Build history of the part. All positions in model axes, mm. Give positions to 0.01 mm unless a question says otherwise; leave off trailing zeros. Write each loop counter-clockwise with the first axis right and the second up, starting at its lowest first coordinate (ties: lowest second). Pieces come first, ordered by that corner, then holes. Notation, with made-up numbers: (-28, 69) -> (-22, 69) arc R16 cw to (-22, 87) -> close; hole circle Ø8 at (-35, 83). An arc over 180 degrees is marked (long way). Write item = value, one per line. Start each with the question number.
Q1. Wall check: line 1 (Z direction, x = 1.65, y = 12.7); line 2 (Y direction, x = 0.55, z = 23); line 3 (Z direction, x = 1.5, y = 45.72). Give the ranges that are in metal, low to high.
Q2. Mould opens along Z. For faces 1 (the face through (2, 55, 38.1)), 2 (the face through (0, 53, 19)), 3 (the face through (1.5, 13.62, 16.82)) say: pulls with the +Z half, pulls with the -Z half, needs draft (parallel to the pull), parting line crosses it, or undercut.
Q3. Drop a flat-ended pin along its axis: P1, Ø1, axis at y = 22.5, z = 6.5, coming from the -X side. Give the stop position or say it passes through.
Q4. Saw through at D-D, the plane z = 19.05. List the corners of the cut face in (x, y).
Q5. Saw through at B-B, the plane x = 2.15. List the corners of the cut face in (y, z).
Q6. Saw through at A-A, the plane z = 6.35. List the corners of the cut face in (x, y).
Q7. Saw through at C-C, the plane y = 45.72. List the corners of the cut face in (x, z).
Autodesk Fusion 360 part; units mm, degrees
sketch "Sketch1" plane through (0, 0, 0) normal (1, 0, 0) x (0, 1, 0)
  line L0 (0, 0) -> (107.95, 0)
  line L1 (107.95, 0) -> (107.95, 38.1)
  line L2 (107.95, 38.1) -> (0, 38.1)
  line L3 (0, 38.1) -> (0, 0)
  dimension "d1" = 38.1
  dimension "d2" = 107.95
extrude "Extrude1" add sketch "Sketch1" along normal blind 3.048
sketch "Sketch2" plane through (3.048, 0, 0) normal (1, 0, 0) x (0, 1, 0)
  line L0 (0, 38.1) -> (0, 0)
  line L1 (0, 0) -> (107.95, 0)
  line L2 (107.95, 0) -> (107.95, 38.1)
  line L3 (107.95, 38.1) -> (0, 38.1)
  line L4 (-12.7, 0) -> (-12.7, 19.05)
  line L5 (0, -12.7) -> (25.4, -12.7)
  line L6 (25.4, -25.4) -> (31.75, -25.4)
  line L7 (33.02, -38.1) -> (45.72, -38.1)
  line L8 (45.72, -50.8) -> (58.42, -50.8)
  line L9 (58.42, -50.8) -> (58.42, -38.1)
  line L10 (58.42, -38.1) -> (71.12, -38.1)
  line L11 (71.12, -38.1) -> (71.12, -50.8)
  line L12 (71.12, -50.8) -> (83.82, -50.8)
  line L13 (83.82, -50.8) -> (83.82, -38.1)
  line L14 (83.82, -38.1) -> (96.52, -38.1)
  line L15 (96.52, -38.1) -> (96.52, -50.8)
  line L16 (96.52, -50.8) -> (109.22, -50.8)
  line L17 (109.22, -50.8) -> (109.22, -38.1)
  line L18 (-12.7, 19.05) -> (121.92, 19.05)
  circle A0 centre (45.72, 19.05) radius 4.826
  dimension "d5" = 19.05
  dimension "d6" = 6.35
  dimension "d7" = 9.652
hole "Hole1" at (3.048, 45.72, 19.05) direction (-1, 0, 0) diameter 9.652 depth 40.64 tip angle 118
sketch "Sketch3" plane through (3.048, 0, 0) normal (1, 0, 0) x (0, 1, 0)
  circle A0 centre (45.72, 19.05) radius 4.826
  line L0 (0, 38.1) -> (0, 0)
  line L1 (0, 0) -> (107.95, 0)
  line L2 (107.95, 0) -> (107.95, 38.1)
  line L3 (107.95, 38.1) -> (0, 38.1)
  line L4 (111.76, 0) -> (111.76, 19.05)
  circle A1 centre (95.25, 19.0673) radius 4.826
  dimension "d16" = 9.652
hole "Hole2" at (3.048, 95.25, 19.0673) direction (-1, 0, 0) diameter 9.652 depth 40.64 tip angle 118
sketch "Sketch4" plane through (3.048, 0, 0) normal (1, 0, 0) x (0, 1, 0)
  circle A0 centre (95.25, 19.0673) radius 4.826
  circle A1 centre (45.72, 19.05) radius 4.826
  line L0 (0, 38.1) -> (0, 0)
  line L1 (0, 0) -> (107.95, 0)
  line L2 (107.95, 0) -> (107.95, 38.1)
  line L3 (107.95, 38.1) -> (0, 38.1)
  line L4 (12.7, -55.88) -> (0, -55.88)
  line L5 (0, -55.88) -> (0, 45.72)
  line L6 (12.7, 0) -> (-25.4, 0)
  line L7 (0, 0) -> (12.7, 0)
  line L8 (12.7, 0) -> (12.7, 6.35)
  line L9 (12.7, 6.35) -> (0, 6.35)
  line L10 (0, 6.35) -> (0, 0)
  dimension "d22" = 12.7
  dimension "d23" = 6.35
hole "Hole3" at (3.048, 12.7, 6.35) direction (-1, 0, 0) diameter 4.826 depth 40.64 tip angle 118
sketch "Sketch5" plane through (3.048, 0, 0) normal (1, 0, 0) x (0, 1, 0)
  circle A0 centre (12.7, 6.35) radius 2.413
  circle A1 centre (95.25, 19.0673) radius 4.826
  circle A2 centre (45.72, 19.05) radius 4.826
  line L0 (0, 38.1) -> (0, 0)
  line L1 (0, 0) -> (107.95, 0)
  line L2 (107.95, 0) -> (107.95, 38.1)
  line L3 (107.95, 38.1) -> (0, 38.1)
  line L4 (0, 38.1) -> (12.7, 38.1)
  line L5 (12.7, 38.1) -> (12.7, 31.75)
  line L6 (12.7, 31.75) -> (0, 31.75)
  line L7 (0, 31.75) -> (0, 38.1)
  dimension "d27" = 12.7
  dimension "d28" = 6.35
hole "Hole4" at (3.048, 12.7, 31.75) direction (-1, 0, 0) diameter 4.826 depth 40.64 tip angle 118
sketch "Sketch6" plane through (3.048, 0, 0) normal (1, 0, 0) x (0, 1, 0)
  circle A0 centre (12.7, 31.75) radius 2.413
  circle A1 centre (12.7, 6.35) radius 2.413
  circle A2 centre (95.25, 19.0673) radius 4.826
  circle A3 centre (45.72, 19.05) radius 4.826
  line L0 (0, 38.1) -> (0, 0)
  line L1 (0, 0) -> (107.95, 0)
  line L2 (107.95, 0) -> (107.95, 38.1)
  line L3 (107.95, 38.1) -> (0, 38.1)
  line L4 (0, 0) -> (12.7, 0)
  line L5 (12.7, 0) -> (12.7, 19.05)
  line L6 (12.7, 19.05) -> (0, 19.05)
  line L7 (0, 19.05) -> (0, 0)
  dimension "d32" = 12.7
  dimension "d33" = 19.05
hole "Hole5" at (3.048, 12.7, 19.05) direction (-1, 0, 0) diameter 4.826 depth 40.64 tip angle 118
Report:
q1.line_1 = 0 to 3.94, 8.76 to 16.64, 21.46 to 29.34, 34.16 to 38.1
q1.line_2 = 0 to 42.95, 48.49 to 92.45, 98.05 to 107.95
q1.line_3 = 0 to 14.22, 23.88 to 38.1
q2.face_1 = pulls with the +Z half
q2.face_2 = needs draft
q2.face_3 = undercut
q3.P1 = 0
q4.outline = (0, 0) -> (3.05, 0) -> (3.05, 10.29) -> (0, 10.29) -> close; (0, 15.11) -> (3.05, 15.11) -> (3.05, 40.89) -> (0, 40.89) -> close; (0, 50.55) -> (3.05, 50.55) -> (3.05, 90.42) -> (0, 90.42) -> close; (0, 100.08) -> (3.05, 100.08) -> (3.05, 107.95) -> (0, 107.95) -> close
q5.outline = (0, 0) -> (107.95, 0) -> (107.95, 38.1) -> (0, 38.1) -> close; hole circle Ø4.83 at (12.7, 6.35); hole circle Ø4.83 at (12.7, 19.05); hole circle Ø4.83 at (12.7, 31.75); hole circle Ø9.65 at (45.72, 19.05); hole circle Ø9.65 at (95.25, 19.07)
q6.outline = (0, 0) -> (3.05, 0) -> (3.05, 10.29) -> (0, 10.29) -> close; (0, 15.11) -> (3.05, 15.11) -> (3.05, 107.95) -> (0, 107.95) -> close
q7.outline = (0, 0) -> (3.05, 0) -> (3.05, 14.22) -> (0, 14.22) -> close; (0, 23.88) -> (3.05, 23.88) -> (3.05, 38.1) -> (0, 38.1) -> close
